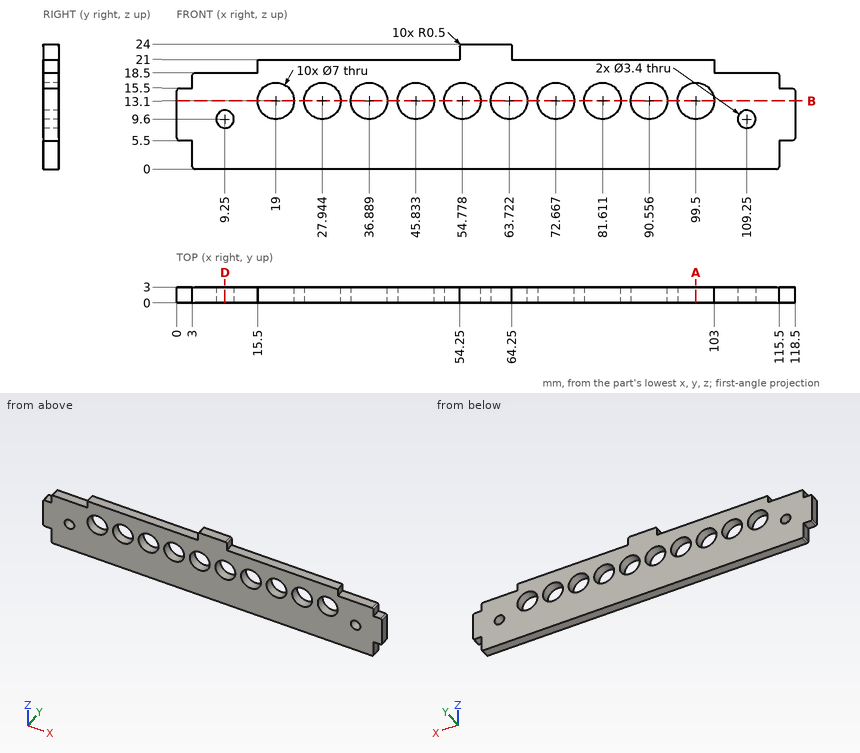
Geometry check sheet. Reference: drawing and pictorial views, mm from the part's lowest x, y, z. Coordinates: 2 decimals unless noted, no trailing zeros. Order: outer loops, then holes, each group sorted by start corner. A loop starts at its lowest first (then second) coordinate and runs counter-clockwise, first axis right, second up. Notation, with made-up numbers: (38.25, -34.75) - (61.25, -34.75) arc R25 ccw to (61.25, -13.75) - close; hole circle Ø8 at (-5, 3). An arc over 180 degrees is marked (long way). One line per item, written item: value.
(1) Sectioned sample at B-B (z = 13.1). Count the separate pieces of the cut face and the enclosed holes in it.
Data:
separate pieces: 11
enclosed holes: 0
(2) Depth check by flat-ended pin: pin 1 Ø1.5 at (y, z) = (1.5, 17) entering from +X; pin 2 Ø0.9 at (x, y) = (107.5, 1.5) entering from +Z; pin 3 Ø11 at (x, z) = (36.89, 13.1) entering from -Y; pin 4 Ø1.2 at (y, z) = (1, 22.5) entering from +X. Enter the tip coordinate at first touch or a pass-through.
Data:
pin 1: stops at x = 115.5
pin 2: stops at z = 18.5
pin 3: stops at y = 0
pin 4: stops at x = 64.25
(3) Sectioned sample at D-D (x = 9.25). Enter the section's corners in (y, z), and give its area (3 significant figures).
Data:
outline: (0, 0) - (3, 0) - (3, 7.9) - (0, 7.9) - close; (0, 11.3) - (3, 11.3) - (3, 18.5) - (0, 18.5) - close
area: 45.3 mm^2
(4) Thickness scan on probe 1 along Z at (x, y) = (109, 2.4); probe 2 along Z at (x, y) = (99.5, 0.7); probe 3 along Z at (x, y) = (50, 1.85). Record the ranges inside material, lowest first. Write a range as from..to.
Data:
probe 1: z = 0..7.92, 11.28..18.5
probe 2: z = 0..9.6, 16.6..21
probe 3: z = 0..21
(5) Sectioned sample at A-A (x = 99.5). Enter the section's corners in (y, z), and give its area (3 significant figures).
Data:
outline: (0, 0) - (3, 0) - (3, 9.6) - (0, 9.6) - close; (0, 16.6) - (3, 16.6) - (3, 21) - (0, 21) - close
area: 42.0 mm^2
